Can you work these out from the model? Positions are in its coordinate system, mm. Give positions to 0.01 mm unless a question says otherwise; leave off trailing zeros. Order: outer loops, then holes, each group sorted by start corner. A loop starts at its lowest first (then second) coordinate and runs counter-clockwise, first axis right, second up. Notation, with made-up numbers: (-36.5, 56) - (-19.5, 56) arc R27 ccw to (-19.5, 75) - close; hole circle Ø9 at (88.25, -30). An arc over 180 degrees is marked (long way). Use one line per item in the form item = value. Start each with the question number.
1) For pin 1 (1.6 mm diameter, centred on x = 10.5, z = -37, fed in from -Y); pin 2 (1.4 mm diameter, centred on x = 10.75, z = -36.72, fed in from -Y); pin 3 (0.8 mm diameter, centred on x = -6, y = -0.5, fed in from +Z), each with a flat end and sliding along its axis, tell me the tip position at first contact or that it passes through.
2) Please list where these lines run through material, in increasing order: probe 1 along Z at (x, y) = (10.75, 4.75); probe 2 along X at (y, z) = (6.75, -29.1); probe 3 along Z at (x, y) = (11, 4).
3) Suppose I cut it at C-C, the plane z = -41.5. Write out the boundary of the cut face in (x, y).
4) Suppose I cut it at A-A, the plane z = -61. Write out the boundary of the cut face in (x, y).
5) Suppose I cut it at B-B, the plane x = -6.5. Write out the boundary of the cut face in (y, z).
6) Suppose I cut it at D-D, the plane x = 4. Write out the boundary of the cut face in (y, z).
```python
from build123d import *

# Parameters (mm, degrees)
SKETCH1_W               = 63.5
SKETCH1_H               = 145.4
BOSS_EXTRUDE1_DEPTH     = 18
CUT_EXTRUDE2_DEPTH      = 82.347111196
CUT_EXTRUDE2_DEPTH_BACK = 8
SKETCH3_R               = 0.75
SKETCH4_W               = 15
SKETCH4_H               = 5.7
BOSS_EXTRUDE2_DEPTH     = 1


with BuildPart() as part:
    # Sketch1 → Boss-Extrude1 (new body)
    with BuildSketch(Plane(origin=(0, 0, 0), x_dir=(1, 0, 0), z_dir=(0, 1, 0))):
        Rectangle(SKETCH1_W, SKETCH1_H)
    extrude(amount=BOSS_EXTRUDE1_DEPTH)

    # Sketch3 → Cut-Extrude2 (cut, two sides: drawn at the far end of the back side and taken through both)
    with BuildSketch(Plane.XZ.offset(-CUT_EXTRUDE2_DEPTH_BACK)):
        with Locations(Location((10.75, -29.1, 0), (0, 0, 90))):
            Circle(SKETCH3_R)
        with Locations(Location((10.75, -31.64, 0), (0, 0, 90))):
            Circle(SKETCH3_R)
        with Locations(Location((10.75, -34.18, 0), (0, 0, 90))):
            Circle(SKETCH3_R)
        with Locations(Location((10.75, -36.72, 0), (0, 0, 90))):
            Circle(SKETCH3_R)
    extrude(amount=CUT_EXTRUDE2_DEPTH + CUT_EXTRUDE2_DEPTH_BACK, mode=Mode.SUBTRACT)

    # Sketch4 → Boss-Extrude2 (add)
    with BuildSketch(Plane.XZ):
        with Locations((-6.85, -60.25)):
            Rectangle(SKETCH4_W, SKETCH4_H)
    extrude(amount=BOSS_EXTRUDE2_DEPTH)


solid = part.part
```
Result sheet:
q1.pin_1 = 0
q1.pin_2 = 8
q1.pin_3 = -57.4
q2.probe_1 = -72.7 to -37.47, -35.97 to -34.93, -33.43 to -32.39, -30.89 to -29.85, -28.35 to 72.7
q2.probe_2 = -31.75 to 10, 11.5 to 31.75
q2.probe_3 = -72.7 to -37.43, -36.01 to -34.89, -33.47 to -32.35, -30.93 to -29.81, -28.39 to 72.7
q3.outline = (-31.75, 0) - (31.75, 0) - (31.75, 18) - (-31.75, 18) - close
q4.outline = (-31.75, 0) - (-14.35, 0) - (-14.35, -1) - (0.65, -1) - (0.65, 0) - (31.75, 0) - (31.75, 18) - (-31.75, 18) - close
q5.outline = (-1, -63.1) - (0, -63.1) - (0, -72.7) - (18, -72.7) - (18, 72.7) - (0, 72.7) - (0, -57.4) - (-1, -57.4) - close
q6.outline = (0, -72.7) - (18, -72.7) - (18, 72.7) - (0, 72.7) - close
